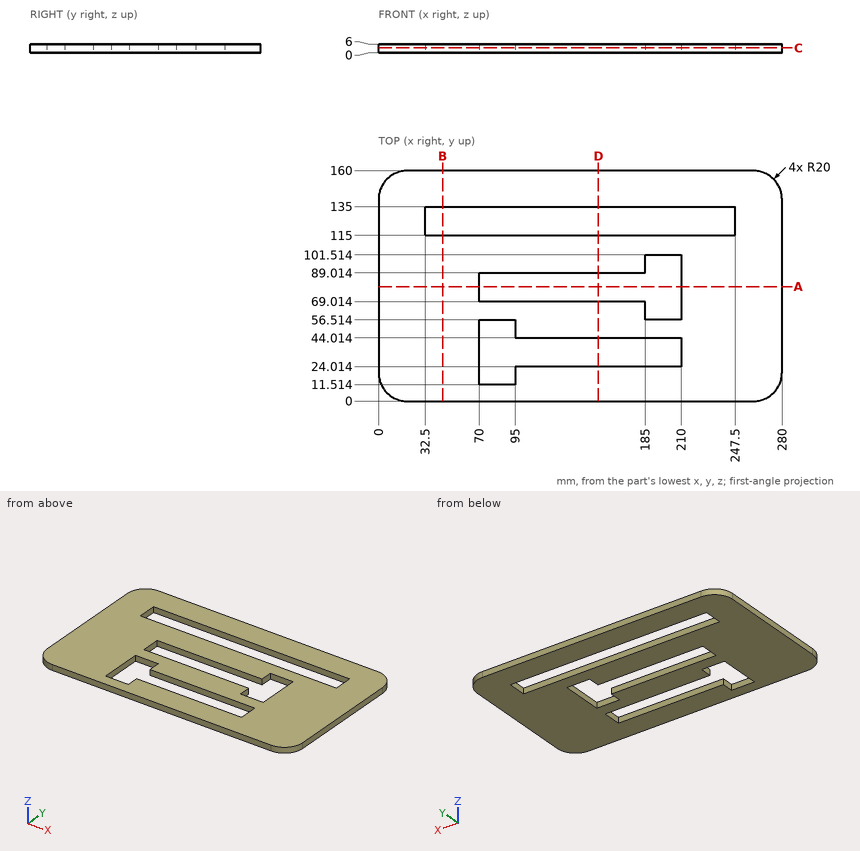
Input: dimensioned drawing with shaded views. Units: mm. Origin: part minimum x, y, z. Coordinates: 2 decimals unless noted, no trailing zeros. Write each loop counter-clockwise with the first axis right and the second up, starting at its lowest first coordinate (ties: lowest second). Pieces come first, ordered by that corner, then holes. Notation, with made-up numbers: (-32, -5) -> (-1, -5) arc R25 ccw to (-1, 28) -> close; hole circle Ø7 at (32.25, 15.5). An arc over 180 degrees is marked (long way). Return JSON: item names as keys, results as strings. Group by question number.
1) Contact query for flat-ended pins moving along their axis: P1, Ø10, axis at x = 154, y = 137, coming from the -Z side; P2, Ø3, axis at y = 143.5, z = 4.5, coming from the -X side; P3, Ø12, axis at x = 77.5, y = 125.5, coming from the +Z side. Output: stop coordinate, or through.
2) Section query C-C, the plane z = 3.25. Return loops of the section in (x, y), plus the area to 3 significant figures.
3) Section query B-B, the plane x = 44.5. Return loops of the section in (y, z).
4) Section query A-A, the plane y = 79.5. Return loops of the section in (x, z), plus the area to 3 significant figures.
5) Ray query, line 1 along Y through (x, z) = (91, 1.7); line 2 along Y through (x, z) = (102.5, 1.8); line 3 along Y through (x, z) = (213, 5.55). Return the intervals inside material, ascending.
6) Section query D-D, the plane x = 152.5. Return loops of the section in (y, z).
From the geometry:
{
 "1": {"P1": "z = 0", "P2": "x = 0.1", "P3": "through"},
 "2": {"outline": "(0, 20) arc R20 ccw to (20, 0) -> (260, 0) arc R20 ccw to (280, 20) -> (280, 140) arc R20 ccw to (260, 160) -> (20, 160) arc R20 ccw to (0, 140) -> close; hole (32.5, 115) -> (247.5, 115) -> (247.5, 135) -> (32.5, 135) -> close; hole (70, 11.51) -> (95, 11.51) -> (95, 24.01) -> (210, 24.01) -> (210, 44.01) -> (95, 44.01) -> (95, 56.51) -> (70, 56.51) -> close; hole (70, 69.01) -> (185, 69.01) -> (185, 56.51) -> (210, 56.51) -> (210, 101.51) -> (185, 101.51) -> (185, 89.01) -> (70, 89.01) -> close", "area": "33,300 mm²"},
 "3": {"outline": "(0, 0) -> (115, 0) -> (115, 6) -> (0, 6) -> close; (135, 0) -> (160, 0) -> (160, 6) -> (135, 6) -> close"},
 "4": {"outline": "(0, 0) -> (70, 0) -> (70, 6) -> (0, 6) -> close; (210, 0) -> (280, 0) -> (280, 6) -> (210, 6) -> close", "area": "840 mm²"},
 "5": {"line 1": "0 to 11.51, 56.51 to 69.01, 89.01 to 115, 135 to 160", "line 2": "0 to 24.01, 44.01 to 69.01, 89.01 to 115, 135 to 160", "line 3": "0 to 115, 135 to 160"},
 "6": {"outline": "(0, 0) -> (24.01, 0) -> (24.01, 6) -> (0, 6) -> close; (44.01, 0) -> (69.01, 0) -> (69.01, 6) -> (44.01, 6) -> close; (89.01, 0) -> (115, 0) -> (115, 6) -> (89.01, 6) -> close; (135, 0) -> (160, 0) -> (160, 6) -> (135, 6) -> close"}
}
